Can you work these out from the model? Positions are in its coordinate system, mm. A direction names the side the tool comes from. Coordinates: 2 decimals unless noted, no trailing zeros. Write each loop counter-clockwise with the first axis right and the second up, starting at its lowest first coordinate (ties: lowest second). Pieces come first, ordered by that corner, then holes.
```python
from build123d import *

# Parameters (mm, degrees)
F0_W     = 63.5
F0_H     = 101.6
F1_DEPTH = 12.7
F2_W     = 25.4
F2_H     = 31.75
F3_DEPTH = 12.7
F5_DEPTH = 12.7


with BuildPart() as f1:
    # F0 (on Top) → F1 (new body)
    with BuildSketch(Plane.XY):
        Rectangle(F0_W, F0_H)
    extrude(amount=F1_DEPTH)

    # F2 (on face) → F3 (join)
    with BuildSketch(Plane.XY.offset(12.7)):
        Polygon((31.75, -50.8), (31.75, 12.7), (12.7, 12.7), (12.7, -19.05), (12.7, -50.8), align=None)
        Polygon((-12.7, -50.8), (-12.7, -19.05), (-12.7, 12.7), (-31.75, 12.7), (-31.75, -50.8), align=None)
        with Locations((0, -34.925)):
            Rectangle(F2_W, F2_H)
    extrude(amount=F3_DEPTH)

    # F4 (on face) → F5 (join)
    with BuildSketch(Plane.XY.offset(25.4)):
        Polygon((-31.75, -50.8), (31.75, -50.8), (31.75, -19.05), (12.7, -19.05), (-12.7, -19.05), (-31.75, -19.05), align=None)
    extrude(amount=F5_DEPTH)


solid = f1.part
```
1. We'd pull the mould along X, two halves only. Please class faces 4 (the face through (-12.7, -3, 19)), 5 (the face through (-22, 12.7, 19)), 6 (the face through (31.75, -12, 15)): released by +X, released by -X, zero draft, split by the parting line, or undercut.
2. If we section it at C-C, the plane y = 25: List the corners of the cut face in (x, z) for me, plus the area to 3 significant figures.
3. If we section it at B-B, the plane x = -16.5: List the corners of the cut face in (y, z) for me, plus the area to 3 significant figures.
4. If I drill on L1, parallel to Z at x = 12, y = 21.5; L2, parallel to Y at x = 25, z = 25.5; L3, parallel to Y at x = -19, z = 20.5, over which ranges is the centre line in solid material (lowest first)?
5. If we section it at A-A, the plane z = 19.5: List the corners of the cut face in (x, y) for me, plus the area to 3 significant figures.
6. I'm going to push flat-ended pins straight in: P1, Ø10, axis at x = -20, z = 20.5, coming from the +Y side; P2, Ø1, axis at x = 1, z = 33.5, coming from the +Y side; P3, Ø1, axis at y = 11.5, z = 26, coming from the -X side; P4, Ø21, axis at x = 21.5, y = -4.5, coming from the +Z side. Where does each tip first touch, or does it pass through?
7. Which directions (+Z, -Z, +X, -X, +Y, -Y) give clear straight access to the entire face, cutting with the end or side of a thin tool? Please do faces 1 (the face through (12.7, -3, 19)), 2 (the face through (0, -50.8, 19)), 3 (the face through (22, 12.7, 19)).
Answers:
1. face 4: undercut
1. face 5: zero draft
1. face 6: released by +X
2. outline: (-31.75, 0) - (31.75, 0) - (31.75, 12.7) - (-31.75, 12.7) - close
2. area: 806 mm2
3. outline: (-50.8, 0) - (50.8, 0) - (50.8, 12.7) - (12.7, 12.7) - (12.7, 25.4) - (-19.05, 25.4) - (-19.05, 38.1) - (-50.8, 38.1) - close
3. area: 2,500 mm2
4. L1: z = 0 to 12.7
4. L2: y = -50.8 to -19.05
4. L3: y = -50.8 to 12.7
5. outline: (-31.75, -50.8) - (31.75, -50.8) - (31.75, 12.7) - (12.7, 12.7) - (12.7, -19.05) - (-12.7, -19.05) - (-12.7, 12.7) - (-31.75, 12.7) - close
5. area: 3,230 mm2
6. P1: stops at y = 12.7
6. P2: stops at y = -19.05
6. P3: passes through
6. P4: stops at z = 25.4
7. face 1: +Z, +Y
7. face 2: +Z, -Z, +X, -X, -Y
7. face 3: +Z, +X, -X, +Y
